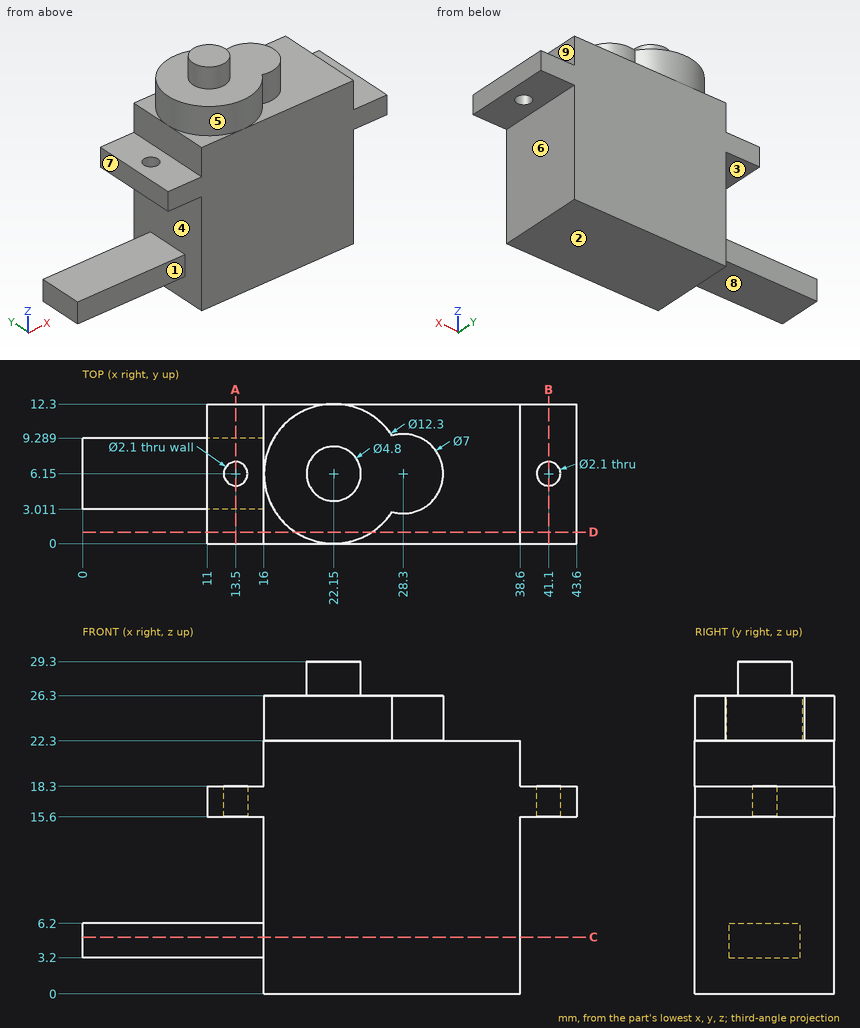
Source: three-view drawing plus pictorial views. Frame: mm from the lowest corner of the part. A direction names the side the tool comes from. Round coordinates to 2 decimals unless told otherwise and drop trailing zeros. Order: outer loops, then holes, each group sorted by start corner. A loop starts at its lowest first (then second) coordinate and runs counter-clockwise, first axis right, second up. Notation, with made-up numbers: (-35.75, -12.75) -> (-22.75, -12.75) arc R23 cw to (-22.75, 24.25) -> close; hole circle Ø3 at (25, -23). An arc over 180 degrees is marked (long way). Use one line per item in the form item = value.
(1) First-contact query: pin 1 Ø8 at (x, z) = (14.5, 3.5) entering from +Y; pin 2 Ø1.9 at (x, y) = (10.5, 5.5) entering from -Z; pin 3 Ø3.5 at (y, z) = (8.5, 10.5) entering from -X; pin 4 Ø2.5 at (x, y) = (13, 5) entering from +Z. Flat tips, straight axial feed; report the tip coordinate or a pass-through.
Results list:
pin_1 = 12.3
pin_2 = 3.2
pin_3 = 16
pin_4 = 18.3
(2) Section A-A on x = 13.5. Return loops of the section in (y, z).
Results list:
outline = (0, 15.6) -> (5.1, 15.6) -> (5.1, 18.3) -> (0, 18.3) -> close; (3.01, 3.2) -> (9.29, 3.2) -> (9.29, 6.2) -> (3.01, 6.2) -> close; (7.2, 15.6) -> (12.3, 15.6) -> (12.3, 18.3) -> (7.2, 18.3) -> close
(3) Section D-D on y = 1. Return loops of the section in (x, z).
Results list:
outline = (11, 15.6) -> (16, 15.6) -> (16, 0) -> (38.6, 0) -> (38.6, 15.6) -> (43.6, 15.6) -> (43.6, 18.3) -> (38.6, 18.3) -> (38.6, 22.3) -> (25.51, 22.3) -> (25.51, 26.3) -> (18.79, 26.3) -> (18.79, 22.3) -> (16, 22.3) -> (16, 18.3) -> (11, 18.3) -> close
(4) Section B-B on x = 41.1. Return loops of the section in (y, z).
Results list:
outline = (0, 15.6) -> (5.1, 15.6) -> (5.1, 18.3) -> (0, 18.3) -> close; (7.2, 15.6) -> (12.3, 15.6) -> (12.3, 18.3) -> (7.2, 18.3) -> close
(5) Access query for the marked faces 5, 6, 7, 8 and 9. Directions: +Z, -Z, +X, -X, +Y, -Y. A direction counts if a zero-diameter tool reaches every point of the face in a straight line with its end or side. Return the directions, or none.
Results list:
face_5 = +Z
face_6 = -Z, +X, +Y, -Y
face_7 = +Z, -X, +Y, -Y
face_8 = -Z, -X, +Y, -Y
face_9 = +Z, +X, +Y, -Y
(6) Ray query, probe 1 along Y at (x, z) = (41.1, 16.25); probe 2 along X at (y, z) = (5, 8); probe 3 along Z at (x, y) = (12.5, 4). Return the intervals inside material, ascending. Write a range as [from, to].
Results list:
probe_1 = [0, 5.1], [7.2, 12.3]
probe_2 = [16, 38.6]
probe_3 = [3.2, 6.2], [15.6, 18.3]
(7) Section C-C on z = 5. Return loops of the section in (x, y), and give its area (3 significant figures).
Results list:
outline = (0, 3.01) -> (16, 3.01) -> (16, 0) -> (38.6, 0) -> (38.6, 12.3) -> (16, 12.3) -> (16, 9.29) -> (0, 9.29) -> close
area = 378 mm^2
(8) Draft query along Z for the marked faces 1, 2, 3 and 4. Return one class per face: pulls with the +Z half, pulls with the -Z half, needs draft (parallel to the pull), parting line crosses it, or undercut.
Results list:
face_1 = needs draft
face_2 = pulls with the -Z half
face_3 = undercut
face_4 = undercut
